For this review, take the finished solid that the model builds, in its own axes (mm). A direction names the side the tool comes from. Round coordinates to 2 decimals unless told otherwise and drop trailing zeros. Order: outer loops, then holes, each group sorted by start corner. A loop starts at its lowest first (then second) coordinate and runs counter-clockwise, first axis right, second up. Notation, with made-up numbers: M 75,4 L 86,4 A28 cw 86,29 Z; hole C -9.5,88 d1. An arc over 180 degrees is marked long. Use a Markdown table: item, result.
from build123d import *

# Parameters (mm, degrees)
SKETCH1_W           = 20
SKETCH1_H           = 10
SKETCH1_W_2         = 17
SKETCH1_H_2         = 7
BOSS_EXTRUDE1_DEPTH = 175
SKETCH2_R           = 1.5
CUT_EXTRUDE1_DEPTH  = 176.570498661
SKETCH3_R           = 2
SKETCH3_R_2         = 3
CUT_EXTRUDE2_DEPTH  = 176.570498661
SKETCH5_R           = 10.770329614
SKETCH5_R_2         = 9.770329614
BOSS_EXTRUDE2_DEPTH = 10


with BuildPart() as part:
    # Sketch1 → Boss-Extrude1 (new body)
    with BuildSketch(Plane.XY):
        Rectangle(SKETCH1_W, SKETCH1_H)
        Rectangle(SKETCH1_W_2, SKETCH1_H_2, mode=Mode.SUBTRACT)
    extrude(amount=BOSS_EXTRUDE1_DEPTH)

    # Sketch2 → Cut-Extrude1 (cut, through all)
    with BuildSketch(Plane(origin=(0, 5, 0), x_dir=(1, 0, 0), z_dir=(0, 1, 0))):
        with Locations(Location((6.363961031, -166.646446609, 0), (0, 0, 180))):
            Circle(SKETCH2_R)
        with Locations(Location((-6.717514421, -167, 0), (0, 0, 180))):
            Circle(SKETCH2_R)
        with Locations(Location((6.717514421, -153.564971157, 0), (0, 0, 180))):
            Circle(SKETCH2_R)
        with Locations(Location((-6.363961031, -153.918524548, 0), (0, 0, 180))):
            Circle(SKETCH2_R)
    extrude(amount=-CUT_EXTRUDE1_DEPTH, mode=Mode.SUBTRACT)

    # Sketch3 → Cut-Extrude2 (cut, through all)
    with BuildSketch(Plane(origin=(0, 5, 0), x_dir=(1, 0, 0), z_dir=(0, 1, 0))):
        with Locations(Location((0, -4, 0), (0, 0, 180))):
            Circle(SKETCH3_R)
        with Locations(Location((0, -24, 0), (0, 0, 180))):
            Circle(SKETCH3_R_2)
    extrude(amount=-CUT_EXTRUDE2_DEPTH, mode=Mode.SUBTRACT)

    # Sketch5 → Boss-Extrude2 (add)
    with BuildSketch(Plane(origin=(0, 5, 0), x_dir=(1, 0, 0), z_dir=(0, 1, 0))):
        with Locations((0, -4)):
            Circle(SKETCH5_R)
        with Locations((0, -4)):
            Circle(SKETCH5_R_2, mode=Mode.SUBTRACT)
    extrude(amount=-BOSS_EXTRUDE2_DEPTH)


solid = part.part
Q1. Add section D-D (y = 0.5). Write out the cut boundary in (x, z), then the cut area to 3 significant figures.
Determined:
| item | result |
|---|---|
| outline | M -10,8 A10.77 ccw long 10,8 L 10,175 L 8.5,175 L 8.5,10.61 A10.77 ccw -8.5,10.61 L -8.5,175 L -10,175 Z; hole M -8.91,0 A9.77 ccw 8.91,0 L 8.5,0 L 8.5,8.82 A9.77 ccw -8.5,8.82 L -8.5,0 Z |
| area | 577 mm^2 |
Q2. Add section A-A (z = 24). Write out the cut boundary in (x, y).
Determined:
| item | result |
|---|---|
| outline | M -10,-5 L -3,-5 L -3,-3.5 L -8.5,-3.5 L -8.5,3.5 L -3,3.5 L -3,5 L -10,5 Z; M 3,-5 L 10,-5 L 10,5 L 3,5 L 3,3.5 L 8.5,3.5 L 8.5,-3.5 L 3,-3.5 Z |
Q3. Clearance check with flat-ended pins moving along their axes: pin 1 (3 mm diameter, centred on y = 1.5, z = 142, fed in from +X); pin 2 (1 mm diameter, centred on y = 3, z = 131, fed in from -X); pin 3 (1.8 mm diameter, centred on x = -6.72, z = 167, fed in from +Y). State where each tip first meets the part, or that it passes through.
Determined:
| item | result |
|---|---|
| pin 1 | stops at x = 10 |
| pin 2 | stops at x = -10 |
| pin 3 | passes through |
Q4. Wall thickness on line 1 along Z through (x, y) = (0, 3.95); line 2 along X through (y, z) = (-2.5, 162); line 3 along Z through (x, y) = (-1, 4.5): over which ranges is each line inside the solid? List them lowest first. Write a range as [from, to].
Determined:
| item | result |
|---|---|
| line 1 | z = [-6.77, -5.77], [0, 2], [6, 21], [27, 175] |
| line 2 | x = [-10, -8.5], [8.5, 10] |
| line 3 | z = [-6.72, -5.72], [0, 2.27], [5.73, 21.17], [26.83, 175] |
Q5. Add section C-C (z = 137.5). Write out the cut boundary in (x, y).
Determined:
| item | result |
|---|---|
| outline | M -10,-5 L 10,-5 L 10,5 L -10,5 Z; hole M -8.5,-3.5 L 8.5,-3.5 L 8.5,3.5 L -8.5,3.5 Z |
Q6. Draft analysis for pull direction Z (two halves, no side actions). For faces 5 (the flat face through (-10, 0, 90)), 6 (the cylindrical face through (0.294, 0.07, -6.766)), 7 (the cylindrical face through (6.559, -4.24, 168.134)), 8 (the cylindrical face through (0, 4, 2)), state which applies: pulls with the +Z half, pulls with the -Z half, needs draft (parallel to the pull), parting line crosses it, or undercut.
Determined:
| item | result |
|---|---|
| face 5 | needs draft |
| face 6 | parting line crosses it |
| face 7 | undercut |
| face 8 | undercut |
Q7. Machinability: for faces 1 (the flat face through (8.5, 0, 4)), 2 (the flat face through (0, 3.5, 92)), 3 (the flat face through (10, 0, 90)), 4 (the cylindrical face through (0.65, 4.26, 21.07)), which of the approach directions +Z, -Z, +X, -X, +Y, -Y give a long, thin tool a straight path to every point of the face, cutting with its end or side? Answer none if there is none.
Determined:
| item | result |
|---|---|
| face 1 | none |
| face 2 | +Z |
| face 3 | +Z, +X, +Y, -Y |
| face 4 | +Y, -Y |
Q8. Add section B-B (x = 0). Give the number of separate pieces and of enclosed holes in the cut face, then the cut area to 3 significant figures.
Determined:
| item | result |
|---|---|
| separate pieces | 6 |
| enclosed holes | 0 |
| area | 512 mm^2 |
